Check sheet for the modelled part. Datum: model origin and axes. Units: mm. A direction names the side the tool comes from. Give positions to 0.01 mm unless a question says otherwise; leave off trailing zeros. Loops run counter-clockwise (first coordinate to the right, second up) from the corner with the lowest first, then second, coordinate; pieces in that order, holes last. Notation, with made-up numbers: (10, 17) -> (33, 17) arc R17 cw to (33, 41) -> close; hole circle Ø6 at (44, 22.5). An arc over 180 degrees is marked (long way). Write each question's results on one line, items separated by ' | '. Start each with the question number.
1. Cross-section at D-D on y = 20. Record the boundary of the cut face in (x, z), and give its area (3 significant figures).
2. Tool access check on faces 1 (the face through (38.486, 0.202, 38.087)), 2 (the face through (-1, 4.55, 50)). Record the directions out of +Z, -Z, +X, -X, +Y, -Y that give a thin tool (end or side, any length) a straight path to the whole face; none if there is none.
3. Cross-section at B-B on x = 11. Record the boundary of the cut face in (y, z).
4. Cross-section at A-A on z = 41.55. Record the boundary of the cut face in (x, y).
5. Cross-section at C-C on x = -29. Record the boundary of the cut face in (y, z), and give its area (3 significant figures).
6. Material ranges on L1, parallel to Y at x = -10, z = 82.5; L2, parallel to Z at x = -5.5, y = -1.5; L3, parallel to Y at x = 5, z = 116, recorded low to high. Write a range as from..to.
7. Mould release check, pull along X, two halves, no side actions. Record for faces 3 (the face through (-39.5, 0, 89)), 4 (the face through (-39, 0, 60)), 5 (the face through (-1, 2, 0)): +X half, -X half, draft (parallel to the pull), parting line (faces both ways), or undercut.
8. Gauge pin test, flat ends, axial feed: pin 1 Ø8 at (x, z) = (-10, 98) entering from +Y; pin 2 Ø2 at (x, y) = (16.5, -22.5) entering from -Z; pin 3 Ø5 at (x, z) = (-23.5, 61) entering from -Y. Record the tip position at first contact, or that the pin passes through.
from build123d import *

# Parameters (mm, degrees)
F0_W         = 79
F0_H         = 9.1
F0_W_2       = 75
F0_H_2       = 5.1
F1_DEPTH     = 100
F0_W_3       = 55
F0_H_3       = 2.1
F2_DEPTH     = 2
F3_R         = 1.55
F4_DEPTH     = 79.001
F6_DEPTH     = 79
F7_DEPTH     = 2
F8_T1_DEPTH  = 5.1
F8_T3_DEPTH  = 79.5142210175
F8_T8_DEPTH  = 65.7327098225
F8_T15_DEPTH = 79.5142210175
F8_T20_DEPTH = 65.7327098225
F8_T28_DEPTH = 65.7327098225
F8_T33_DEPTH = 79.5142210175


# Not quite as in the source:
# - a fillet or chamfer that OpenCascade refuses, or shapes differently, is made with other operations: its cross-section is extruded or revolved along the edge and cut away or added


with BuildPart() as f1:
    # F0 (on Top) → F1 (new body)
    with BuildSketch(Plane.XY):
        Rectangle(F0_W, F0_H)
        Rectangle(F0_W_2, F0_H_2, mode=Mode.SUBTRACT)
    extrude(amount=F1_DEPTH)

    # F0 (on Top) → F2 (join)
    with BuildSketch(Plane.XY):
        Rectangle(F0_W, F0_H)
        Rectangle(F0_W_2, F0_H_2, mode=Mode.SUBTRACT)
        Rectangle(F0_W_2, F0_H_2)
        Rectangle(F0_W_3, F0_H_3, mode=Mode.SUBTRACT)
    extrude(amount=-F2_DEPTH)

    # F3 (on face) → F4 (cut, through all)
    with BuildSketch(Plane(origin=(-39.5, 0, 0), x_dir=(0, -1, 0), z_dir=(-1, 0, 0))):
        with BuildLine():
            ThreePointArc((0, 0), (1.0960155108, 0.4539844892), (1.55, 1.55))
            ThreePointArc((1.55, 1.55), (-1.0960155108, 2.6460155108), (0, 0))
        make_face()
        with Locations((0, 6.55)):
            Circle(F3_R)
        with Locations((0, 11.55)):
            Circle(F3_R)
        with Locations((0, 16.55)):
            Circle(F3_R)
        with Locations((0, 21.55)):
            Circle(F3_R)
        with Locations((0, 26.55)):
            Circle(F3_R)
        with Locations((0, 31.55)):
            Circle(F3_R)
        with Locations((0, 36.55)):
            Circle(F3_R)
        with Locations((0, 41.55)):
            Circle(F3_R)
        with Locations((0, 46.55)):
            Circle(F3_R)
        with Locations((0, 51.55)):
            Circle(F3_R)
        with Locations((0, 56.55)):
            Circle(F3_R)
        with Locations((0, 61.55)):
            Circle(F3_R)
        with Locations((0, 66.55)):
            Circle(F3_R)
        with Locations((0, 71.55)):
            Circle(F3_R)
        with Locations((0, 76.55)):
            Circle(F3_R)
        with Locations((0, 81.55)):
            Circle(F3_R)
        with Locations((0, 86.55)):
            Circle(F3_R)
        with Locations((0, 91.55)):
            Circle(F3_R)
        with Locations((0, 96.55)):
            Circle(F3_R)
    extrude(amount=-F4_DEPTH, mode=Mode.SUBTRACT)

    # F5 (on face) → F6 (join, through all)
    with BuildSketch(Plane(origin=(-39.5, 0, 0), x_dir=(0, -1, 0), z_dir=(-1, 0, 0))):
        Polygon((-29.7229889353, 130), (-4.55, 100), (-2.55, 100), (-27.7229889353, 130), align=None)
        Polygon((27.7229889353, 130), (2.55, 100), (4.55, 100), (29.7229889353, 130), align=None)
    extrude(amount=-F6_DEPTH)

    # F5 (on face) → F7 (join, through all)
    with BuildSketch(Plane(origin=(-39.5, 0, 0), x_dir=(0, -1, 0), z_dir=(-1, 0, 0))):
        Polygon((-27.7229889353, 130), (-2.55, 100), (2.55, 100), (27.7229889353, 130), align=None)
    extrude(amount=-F7_DEPTH)

    # F8: chamfer of 2 on 4 edges, made by hand

    # F8_s2 → F8_t1 (cut)
    with BuildSketch(Plane.XZ.offset(-2.55)):
        Polygon((37.5, 98), (39.5, 100), (37.5, 100), align=None)
    extrude(amount=F8_T1_DEPTH, mode=Mode.SUBTRACT)

    # F8_s4 → F8_t3 (cut)
    with BuildSketch(Plane.YZ.offset(-37.5)):
        Polygon((-28.6556042516, 130), (-27.1235153654, 129.2855752194), (-27.7229889353, 130), align=None)
        Polygon((28.6556042516, 130), (27.1235153654, 129.2855752194), (27.7229889353, 130), align=None)
    extrude(amount=F8_T3_DEPTH, mode=Mode.SUBTRACT)


with BuildPart() as f8_tool6:
    # F8_s7 → F8_t8 (new body)
    with BuildSketch(Plane.XZ.offset(32.8663549113)):
        Polygon((-39.5, 130), (-37.5, 128), (-37.5, 130), align=None)
    extrude(amount=-F8_T8_DEPTH)

    split(bisect_by=Plane(origin=(0, -47.7439862241, 40.0619612316), x_dir=(1, 0, 0), z_dir=(0, -0.7660444431, 0.6427876097)), keep=Keep.TOP)

    split(bisect_by=Plane(origin=(0, 47.7439862241, 40.0619612316), x_dir=(1, 0, 0), z_dir=(0, 0.7660444431, 0.6427876097)), keep=Keep.TOP)


with BuildPart() as f1_1:
    add(f1.part)

    # F8_t5: cut F8_tool6
    add(f8_tool6.part, mode=Mode.SUBTRACT)


with BuildPart() as f8_tool13:
    # F8_s14 → F8_t15 (new body)
    with BuildSketch(Plane.YZ.offset(-40.0142210175)):
        Polygon((-28.6556042516, 130), (-27.1235153654, 129.2855752194), (-27.7229889353, 130), align=None)
    extrude(amount=F8_T15_DEPTH)

    split(bisect_by=Plane.YZ.offset(-37.5), keep=Keep.BOTTOM)

    split(bisect_by=Plane.YZ.offset(-39.5), keep=Keep.TOP)


with BuildPart() as f8_tool18:
    # F8_s19 → F8_t20 (new body)
    with BuildSketch(Plane.XZ.offset(32.8663549113)):
        Polygon((-39.5, 130), (-37.5, 128), (-37.5, 130), align=None)
    extrude(amount=-F8_T20_DEPTH)

    split(bisect_by=Plane(origin=(0, 46.5703380464, 39.0771534786), x_dir=(1, 0, 0), z_dir=(0, 0.7660444431, 0.6427876097)), keep=Keep.TOP)

    split(bisect_by=Plane(origin=(0, 47.7439862241, 40.0619612316), x_dir=(1, 0, 0), z_dir=(0, -0.7660444431, -0.6427876097)), keep=Keep.TOP)


with BuildPart() as f8_tool13_1:
    add(f8_tool13.part)

    # F8_t23: intersect F8_tool18
    add(f8_tool18.part, mode=Mode.INTERSECT)


with BuildPart() as f1_2:
    add(f1_1.part)

    # F8_t11: cut F8_tool13
    add(f8_tool13_1.part, mode=Mode.SUBTRACT)


with BuildPart() as f8_tool26:
    # F8_s27 → F8_t28 (new body)
    with BuildSketch(Plane.XZ.offset(32.8663549113)):
        Polygon((-39.5, 130), (-37.5, 128), (-37.5, 130), align=None)
    extrude(amount=-F8_T28_DEPTH)

    split(bisect_by=Plane(origin=(0, -47.7439862241, 40.0619612316), x_dir=(1, 0, 0), z_dir=(0, 0.7660444431, -0.6427876097)), keep=Keep.TOP)

    split(bisect_by=Plane(origin=(0, -46.5703380464, 39.0771534786), x_dir=(1, 0, 0), z_dir=(0, -0.7660444431, 0.6427876097)), keep=Keep.TOP)


with BuildPart() as f8_tool31:
    # F8_s32 → F8_t33 (new body)
    with BuildSketch(Plane.YZ.offset(-40.0142210175)):
        Polygon((28.6556042516, 130), (27.1235153654, 129.2855752194), (27.7229889353, 130), align=None)
    extrude(amount=F8_T33_DEPTH)

    split(bisect_by=Plane.YZ.offset(-37.5), keep=Keep.BOTTOM)

    split(bisect_by=Plane.YZ.offset(-39.5), keep=Keep.TOP)


with BuildPart() as f8_tool26_1:
    add(f8_tool26.part)

    # F8_t36: intersect F8_tool31
    add(f8_tool31.part, mode=Mode.INTERSECT)


with BuildPart() as f1_3:
    add(f1_2.part)

    # F8_t24: cut F8_tool26
    add(f8_tool26_1.part, mode=Mode.SUBTRACT)


solid = f1_3.part
Geometry says:
1) outline: (-39.5, 118.41) -> (39.5, 118.41) -> (39.5, 120.8) -> (-37.5, 120.8) -> (-37.5, 128) -> (-39.5, 130) -> close | area: 205 mm^2
2) face 1: +X, -X | face 2: -Z, +X, -X, +Y
3) outline: (-29.72, 130) -> (-4.55, 100) -> (-4.55, -2) -> (-1.05, -2) -> (-1.05, 0) -> (-2.55, 0) -> (-2.55, 100) -> (-27.12, 129.29) -> (-28.66, 130) -> close; (1.05, -2) -> (4.55, -2) -> (4.55, 100) -> (29.72, 130) -> (28.66, 130) -> (27.12, 129.29) -> (2.55, 100) -> (2.55, 0) -> (1.05, 0) -> close
4) outline: (-39.5, -4.55) -> (39.5, -4.55) -> (39.5, -1.55) -> (37.5, -1.55) -> (37.5, -2.55) -> (-37.5, -2.55) -> (-37.5, -1.55) -> (-39.5, -1.55) -> close; (-39.5, 1.55) -> (-37.5, 1.55) -> (-37.5, 2.55) -> (37.5, 2.55) -> (37.5, 1.55) -> (39.5, 1.55) -> (39.5, 4.55) -> (-39.5, 4.55) -> close
5) outline: (-29.72, 130) -> (-4.55, 100) -> (-4.55, -2) -> (4.55, -2) -> (4.55, 100) -> (29.72, 130) -> (28.66, 130) -> (27.12, 129.29) -> (2.55, 100) -> (2.55, 0) -> (-2.55, 0) -> (-2.55, 100) -> (-27.12, 129.29) -> (-28.66, 130) -> close | area: 538 mm^2
6) L1: -4.55..-2.55, 2.55..4.55 | L2: -2..0 | L3: -17.98..-15.98, 15.98..17.98
7) face 3: -X half | face 4: draft | face 5: undercut
8) pin 1: y = 6.23 | pin 2: z = 120.2 | pin 3: y = -4.55
